from build123d import *

# Parameters (mm, degrees)
F0_R     = 1
F1_DEPTH = 16
F2_T     = -2.5
F3_DEPTH = 8
F4_W     = 41.64
F4_H     = 10.8
F4_W_2   = 11.5
F4_H_2   = 11.5
F4_R     = 2.75
F5_DEPTH = 2.501
F6_SIZE  = 1
F7_SIZE  = 0.5


with BuildPart() as f1:
    # F0 (on Top) → F1 (new body)
    with BuildSketch(Plane.XY):
        with BuildLine():
            ThreePointArc((-36.115, -24.13), (-33.9065851301, -29.4615851301), (-28.575, -31.67))
            Line((-28.575, -31.67), (-26.035, -31.67))
            Line((-26.035, -31.67), (-26.035, -24.13))
            ThreePointArc((-26.035, -24.13), (-26.7789487758, -22.3339487758), (-28.575, -21.59))
            Line((-28.575, -21.59), (-36.115, -21.59))
            Line((-36.115, -21.59), (-36.115, -24.13))
        make_face()
        with Locations((-28.575, -24.13)):
            Circle(F0_R, mode=Mode.SUBTRACT)
        with BuildLine():
            Line((-26.035, -24.13), (-26.035, -31.67))
            Line((-26.035, -31.67), (26.035, -31.67))
            Line((26.035, -31.67), (26.035, -24.13))
            ThreePointArc((26.035, -24.13), (26.7789487758, -22.3339487758), (28.575, -21.59))
            Line((28.575, -21.59), (36.115, -21.59))
            Line((36.115, -21.59), (36.115, 21.59))
            Line((36.115, 21.59), (28.575, 21.59))
            ThreePointArc((28.575, 21.59), (26.7789487758, 22.3339487758), (26.035, 24.13))
            Line((26.035, 24.13), (26.035, 31.67))
            Line((26.035, 31.67), (-26.035, 31.67))
            Line((-26.035, 31.67), (-26.035, 24.13))
            ThreePointArc((-26.035, 24.13), (-26.7789487758, 22.3339487758), (-28.575, 21.59))
            Line((-28.575, 21.59), (-36.115, 21.59))
            Line((-36.115, 21.59), (-36.115, -21.59))
            Line((-36.115, -21.59), (-28.575, -21.59))
            ThreePointArc((-28.575, -21.59), (-26.7789487758, -22.3339487758), (-26.035, -24.13))
        make_face()
        with BuildLine():
            Line((-36.115, 24.13), (-36.115, 21.59))
            Line((-36.115, 21.59), (-28.575, 21.59))
            ThreePointArc((-28.575, 21.59), (-26.7789487758, 22.3339487758), (-26.035, 24.13))
            Line((-26.035, 24.13), (-26.035, 31.67))
            Line((-26.035, 31.67), (-28.575, 31.67))
            ThreePointArc((-28.575, 31.67), (-33.9065851301, 29.4615851301), (-36.115, 24.13))
        make_face()
        with Locations((-28.575, 24.13)):
            Circle(F0_R, mode=Mode.SUBTRACT)
        with BuildLine():
            Line((26.035, -24.13), (26.035, -31.67))
            Line((26.035, -31.67), (28.575, -31.67))
            ThreePointArc((28.575, -31.67), (33.9065851301, -29.4615851301), (36.115, -24.13))
            Line((36.115, -24.13), (36.115, -21.59))
            Line((36.115, -21.59), (28.575, -21.59))
            ThreePointArc((28.575, -21.59), (26.7789487758, -22.3339487758), (26.035, -24.13))
        make_face()
        with Locations((28.575, -24.13)):
            Circle(F0_R, mode=Mode.SUBTRACT)
        with BuildLine():
            Line((28.575, 21.59), (36.115, 21.59))
            Line((36.115, 21.59), (36.115, 24.13))
            ThreePointArc((36.115, 24.13), (33.9065851301, 29.4615851301), (28.575, 31.67))
            Line((28.575, 31.67), (26.035, 31.67))
            Line((26.035, 31.67), (26.035, 24.13))
            ThreePointArc((26.035, 24.13), (26.7789487758, 22.3339487758), (28.575, 21.59))
        make_face()
        with Locations((28.575, 24.13)):
            Circle(F0_R, mode=Mode.SUBTRACT)
        with Locations((28.575, -24.13)):
            Circle(F0_R)
        with Locations((28.575, 24.13)):
            Circle(F0_R)
        with Locations((-28.575, -24.13)):
            Circle(F0_R)
        with Locations((-28.575, 24.13)):
            Circle(F0_R)
    extrude(amount=F1_DEPTH)

    # F2
    f2_openings = [f1.faces().sort_by_distance(p)[0] for p in [
        (0, 0, 16),
    ]]
    offset(amount=F2_T, openings=f2_openings)

    # F0 (on Top) → F3 (join)
    with BuildSketch(Plane.XY):
        with BuildLine():
            Line((26.035, -24.13), (26.035, -31.67))
            Line((26.035, -31.67), (28.575, -31.67))
            ThreePointArc((28.575, -31.67), (33.9065851301, -29.4615851301), (36.115, -24.13))
            Line((36.115, -24.13), (36.115, -21.59))
            Line((36.115, -21.59), (28.575, -21.59))
            ThreePointArc((28.575, -21.59), (26.7789487758, -22.3339487758), (26.035, -24.13))
        make_face()
        with Locations((28.575, -24.13)):
            Circle(F0_R, mode=Mode.SUBTRACT)
        with BuildLine():
            Line((28.575, 21.59), (36.115, 21.59))
            Line((36.115, 21.59), (36.115, 24.13))
            ThreePointArc((36.115, 24.13), (33.9065851301, 29.4615851301), (28.575, 31.67))
            Line((28.575, 31.67), (26.035, 31.67))
            Line((26.035, 31.67), (26.035, 24.13))
            ThreePointArc((26.035, 24.13), (26.7789487758, 22.3339487758), (28.575, 21.59))
        make_face()
        with Locations((28.575, 24.13)):
            Circle(F0_R, mode=Mode.SUBTRACT)
        with BuildLine():
            Line((-36.115, 24.13), (-36.115, 21.59))
            Line((-36.115, 21.59), (-28.575, 21.59))
            ThreePointArc((-28.575, 21.59), (-26.7789487758, 22.3339487758), (-26.035, 24.13))
            Line((-26.035, 24.13), (-26.035, 31.67))
            Line((-26.035, 31.67), (-28.575, 31.67))
            ThreePointArc((-28.575, 31.67), (-33.9065851301, 29.4615851301), (-36.115, 24.13))
        make_face()
        with Locations((-28.575, 24.13)):
            Circle(F0_R, mode=Mode.SUBTRACT)
        with BuildLine():
            ThreePointArc((-36.115, -24.13), (-33.9065851301, -29.4615851301), (-28.575, -31.67))
            Line((-28.575, -31.67), (-26.035, -31.67))
            Line((-26.035, -31.67), (-26.035, -24.13))
            ThreePointArc((-26.035, -24.13), (-26.7789487758, -22.3339487758), (-28.575, -21.59))
            Line((-28.575, -21.59), (-36.115, -21.59))
            Line((-36.115, -21.59), (-36.115, -24.13))
        make_face()
        with Locations((-28.575, -24.13)):
            Circle(F0_R, mode=Mode.SUBTRACT)
    extrude(amount=F3_DEPTH)

    # F4 (on face) → F5 (cut, through all)
    with BuildSketch(Plane.XY.offset(2.5)):
        with Locations((0.365, -19.16)):
            Rectangle(F4_W, F4_H)
        with Locations((-18.415, 13.97)):
            Rectangle(F4_W_2, F4_H_2)
        with Locations((-5.715, 13.97)):
            Circle(F4_R)
        with Locations((-18.415, -6.35)):
            Rectangle(F4_W_2, F4_H_2)
        with Locations((-5.715, -6.35)):
            Circle(F4_R)
        with Locations((13.335, 13.97)):
            Rectangle(F4_W_2, F4_H_2)
        with Locations((26.035, 13.97)):
            Circle(F4_R)
        with Locations((13.335, -6.35)):
            Rectangle(F4_W_2, F4_H_2)
        with Locations((26.035, -6.35)):
            Circle(F4_R)
    extrude(amount=-F5_DEPTH, mode=Mode.SUBTRACT)

    # F6
    f6_edges = [f1.edges().sort_by_distance(p)[0] for p in [
        (-36.115, 0, 16),
        (-33.906585, -29.461585, 16),
        (0, -31.67, 16),
        (33.906585, -29.461585, 16),
        (36.115, 0, 16),
        (33.906585, 29.461585, 16),
        (0, 31.67, 16),
        (-33.906585, 29.461585, 16),
    ]]
    chamfer(f6_edges, length=F6_SIZE)

    # F7
    f7_edges = [f1.edges().sort_by_distance(p)[0] for p in [
        (-33.615, 22.86, 8),
        (-32.138818, 27.693818, 8),
        (-27.305, 29.17, 8),
        (-26.035, 26.65, 8),
        (-26.778949, 22.333949, 8),
        (-31.095, 21.59, 8),
        (-29.575, 24.13, 8),
        (26.778949, 22.333949, 8),
        (26.035, 26.65, 8),
        (27.305, 29.17, 8),
        (32.138818, 27.693818, 8),
        (33.615, 22.86, 8),
        (31.095, 21.59, 8),
        (27.575, 24.13, 8),
        (26.778949, -22.333949, 8),
        (31.095, -21.59, 8),
        (33.615, -22.86, 8),
        (32.138818, -27.693818, 8),
        (27.305, -29.17, 8),
        (26.035, -26.65, 8),
        (27.575, -24.13, 8),
        (-31.095, -21.59, 8),
        (-26.778949, -22.333949, 8),
        (-26.035, -26.65, 8),
        (-27.305, -29.17, 8),
        (-32.138818, -27.693818, 8),
        (-33.615, -22.86, 8),
        (-29.575, -24.13, 8),
        (-26.035, -26.65, 2.5),
        (-26.778949, -22.333949, 2.5),
        (0, -29.17, 2.5),
        (-31.095, -21.59, 2.5),
        (26.035, -26.65, 2.5),
        (-33.615, 0, 2.5),
        (26.778949, -22.333949, 2.5),
        (-31.095, 21.59, 2.5),
        (31.095, -21.59, 2.5),
        (-26.778949, 22.333949, 2.5),
        (33.615, 0, 2.5),
        (-26.035, 26.65, 2.5),
        (31.095, 21.59, 2.5),
        (0, 29.17, 2.5),
        (26.778949, 22.333949, 2.5),
        (26.035, 26.65, 2.5),
        (0.365, -13.76, 2.5),
        (-20.455, -19.16, 2.5),
        (0.365, -24.56, 2.5),
        (21.185, -19.16, 2.5),
        (-12.665, -6.35, 2.5),
        (-18.415, -0.6, 2.5),
        (-24.165, -6.35, 2.5),
        (-18.415, -12.1, 2.5),
        (-8.465, -6.35, 2.5),
        (13.335, -12.1, 2.5),
        (19.085, -6.35, 2.5),
        (13.335, -0.6, 2.5),
        (7.585, -6.35, 2.5),
        (23.285, -6.35, 2.5),
        (-12.665, 13.97, 2.5),
        (-18.415, 19.72, 2.5),
        (-24.165, 13.97, 2.5),
        (-18.415, 8.22, 2.5),
        (-8.465, 13.97, 2.5),
        (13.335, 8.22, 2.5),
        (19.085, 13.97, 2.5),
        (13.335, 19.72, 2.5),
        (7.585, 13.97, 2.5),
        (23.285, 13.97, 2.5),
        (-33.615, 21.59, 5.25),
        (-33.615, -21.59, 5.25),
        (26.035, 29.17, 5.25),
        (-26.035, 29.17, 5.25),
        (33.615, -21.59, 5.25),
        (33.615, 21.59, 5.25),
        (-26.035, -29.17, 5.25),
        (26.035, -29.17, 5.25),
    ]]
    chamfer(f7_edges, length=F7_SIZE)


solid = f1.part
Here's how the part is built. I have some questions about the finished solid (model axes, mm). A direction names the side the tool comes from. Coordinates: 2 decimals unless noted, no trailing zeros. Write each loop counter-clockwise with the first axis right and the second up, starting at its lowest first coordinate (ties: lowest second). Pieces come first, ordered by that corner, then holes.
Item 1: I want a section at C-C on y = -19. Write out the boundary of the cut face in (x, z) (3 decimals).
Item 2: If I drill on line 1 (X direction, y = -24.13, z = 3.85) (3 decimals); line 2 (Y direction, x = -16.5, z = 1.75); line 3 (Y direction, x = 24.5, z = 3.25), over which ranges is the centre line in solid material (lowest first)?
Item 3: Will these pins go through, and if not, where does the flat tip stop? pin 1 (1.3 mm diameter, centred on x = -31.5, z = 5, fed in from +Y); pin 2 (1 mm diameter, centred on x = 28, y = 24.5, fed in from +Z); pin 3 (10 mm diameter, centred on x = 22, y = 5, fed in from +Z).
Item 4: If we mould it in two halves opening along Y, with no side actions, what happens to faces 1 (the cylindrical face through (33.85, -29.52, 7.4)), 2 (the cylindrical face through (-32.18, -27.65, 12.2)), 3 (the flat face through (-36.115, 0, 7))? For each: +Y half, -Y half, draft (parallel to the pull), parting line (faces both ways), or undercut.
Item 5: On a 3-axis mill with a long thin cutter (end or side, diameter ignored), from which of +Z, -Z, +X, -X, +Y, -Y can I reach the whole of each face in a straight line? I mean faces 4 (the cylindrical face through (28.44, -23.14, 4.96)), 5 (the flat face through (13, -12.1, 1)), 6 (the flat face through (0, 31.67, 7)). Say none if no direction works.
Item 6: I want a section at B-B on x = -18.5. Count the separate pieces of the cut face and the enclosed holes in it, and give its area (3 significant figures).
Item 7: I want a section at A-A on z = 10.75. Write out the boundary of the cut face in (x, y) (3 decimals).
Findings below:
1. outline: (-36.115, 0) - (-20.455, 0) - (-20.455, 2) - (-20.955, 2.5) - (-33.115, 2.5) - (-33.615, 3) - (-33.615, 16) - (-35.115, 16) - (-36.115, 15) - close; (21.185, 0) - (36.115, 0) - (36.115, 15) - (35.115, 16) - (33.615, 16) - (33.615, 3) - (33.115, 2.5) - (21.685, 2.5) - (21.185, 2) - close
2. line 1: x = -36.115 to -29.575, -27.575 to -26.035, 26.035 to 27.575, 29.575 to 36.115
2. line 2: y = -31.67 to -24.56, -13.76 to -12.1, -0.6 to 8.22, 19.72 to 31.67
2. line 3: y = -31.67 to -29.17, 29.17 to 31.67
3. pin 1: stops at y = 31.32
3. pin 2: stops at z = 7.68
3. pin 3: stops at z = 2.5
4. face 1: -Y half
4. face 2: undercut
4. face 3: draft
5. face 4: +Z
5. face 5: +Z, -Z
5. face 6: +Z, -Z, +X, -X, +Y
6. separate pieces: 4
6. enclosed holes: 0
6. area: 140 mm2
7. outline: (-36.115, -24.13) arc R7.54 ccw to (-28.575, -31.67) - (28.575, -31.67) arc R7.54 ccw to (36.115, -24.13) - (36.115, 24.13) arc R7.54 ccw to (28.575, 31.67) - (-28.575, 31.67) arc R7.54 ccw to (-36.115, 24.13) - close; hole (-33.615, -24.13) arc R5.04 ccw to (-28.575, -29.17) - (28.575, -29.17) arc R5.04 ccw to (33.615, -24.13) - (33.615, 24.13) arc R5.04 ccw to (28.575, 29.17) - (-28.575, 29.17) arc R5.04 ccw to (-33.615, 24.13) - close
